from build123d import *

# Parameters (mm, degrees)
SKETCH_1_W               = 25
SKETCH_1_H               = 10
EXTRUDE_1_DEPTH          = 22.5
SKETCH_2_W               = 25
SKETCH_2_H               = 15.2
CUT_EXTRUDE_1_DEPTH      = 7.5
CUT_EXTRUDE_2_DEPTH      = 36.089172119
CUT_EXTRUDE_2_DEPTH_BACK = 36.089172119
SKETCH_4_R               = 1.03
SKETCH_5_W               = 25
SKETCH_5_H               = 4.5
EXTRUDE_2_DEPTH          = 20
SKETCH_6_W               = 11
SKETCH_6_H               = 2
CUT_EXTRUDE_3_DEPTH      = 4.5
EXTRUDE_3_DEPTH          = 3.5
SKETCH_16_R              = 9
EXTRUDE_4_DEPTH          = 6
FILLET_1_R               = 3
CUT_EXTRUDE_4_REACH      = 94.322
SKETCH_17_R              = 1.1
SKETCH_19_W              = 13
SKETCH_19_H              = 15.1
CUT_EXTRUDE_5_DEPTH      = 10
EXTRUDE_5_REACH          = 95.01
CUT_EXTRUDE_6_REACH      = 96.037
SKETCH_22_W              = 7
SKETCH_22_H              = 5
FILLET_3_R               = 2


with BuildPart() as part:
    # 草图1 → 凸台-拉伸1 (new body)
    with BuildSketch(Plane(origin=(0, 0, 0), x_dir=(1, 0, 0), z_dir=(0, 1, 0))):
        with Locations((12.5, -5)):
            Rectangle(SKETCH_1_W, SKETCH_1_H)
    extrude(amount=EXTRUDE_1_DEPTH)

    # 草图2 → 切除-拉伸1 (cut)
    with BuildSketch(Plane.XY.offset(10)):
        with Locations((12.5, 10.5)):
            Rectangle(SKETCH_2_W, SKETCH_2_H)
    extrude(amount=-CUT_EXTRUDE_1_DEPTH, mode=Mode.SUBTRACT)

    # 草图4 → 切除-拉伸2 (cut, two sides: drawn at the far end of the back side and taken through both)
    with BuildSketch(Plane(origin=(0, 22.5, 0), x_dir=(1, 0, 0), z_dir=(0, 1, 0)).offset(-CUT_EXTRUDE_2_DEPTH_BACK)):
        with Locations(Location((12.5, -5.7, 0), (0, 0, 270))):
            Circle(SKETCH_4_R)
        with Locations(Location((19.5, -5.7, 0), (0, 0, 270))):
            Circle(SKETCH_4_R)
        with Locations(Location((5.5, -5.7, 0), (0, 0, 270))):
            Circle(SKETCH_4_R)
    extrude(amount=CUT_EXTRUDE_2_DEPTH + CUT_EXTRUDE_2_DEPTH_BACK, mode=Mode.SUBTRACT)

    # 草图5 → 凸台-拉伸2 (add)
    with BuildSketch(Plane(origin=(0, 0, 0), x_dir=(-1, 0, 0), z_dir=(0, 0, -1))):
        with Locations((-12.5, 20.25)):
            Rectangle(SKETCH_5_W, SKETCH_5_H)
    extrude(amount=EXTRUDE_2_DEPTH)

    # 草图6 → 切除-拉伸3 (cut)
    with BuildSketch(Plane(origin=(0, 22.5, 0), x_dir=(1, 0, 0), z_dir=(0, 1, 0))):
        with Locations((12.5, 16)):
            Rectangle(SKETCH_6_W, SKETCH_6_H)
        with Locations((12.5, 4)):
            Rectangle(SKETCH_6_W, SKETCH_6_H)
    extrude(amount=-CUT_EXTRUDE_3_DEPTH, mode=Mode.SUBTRACT)

    # 草图15 → 凸台-拉伸3 (add)
    with BuildSketch(Plane(origin=(0, 22.5, 0), x_dir=(1, 0, 0), z_dir=(0, 1, 0))):
        Polygon((25, -2.5), (50, 11.93375673), (75, -2.5), (75, 17.5), (49.967235844, 31.914840335), (25, 17.5), align=None)
    extrude(amount=-EXTRUDE_3_DEPTH)

    # 草图16 → 凸台-拉伸4 (add)
    with BuildSketch(Plane.XZ.offset(-19)):
        with Locations(Location((75.52146997, -8.282050808, 0), (0, 0, 270))):
            Circle(SKETCH_16_R)
    extrude(amount=-EXTRUDE_4_DEPTH)

    # 圆角1
    # the kernel refuses this fillet: 3 mm, written as the material it adds along each edge
    with BuildSketch(Plane(origin=(50, 22.5, -11.93375673), x_dir=(-0.8660254037844394, 0, 0.4999999999999987), z_dir=(0, -1, 0))) as fillet_1_piece_1:
        with BuildLine():
            CenterArc((FILLET_1_R * 0.57735026919, -FILLET_1_R), FILLET_1_R, 90, 60)
            Line((-FILLET_1_R * 0.288675134595, -FILLET_1_R * 0.5), (-FILLET_1_R * 0.305995642671, -FILLET_1_R * 0.49))
            Line((-FILLET_1_R * 0.305995642671, -FILLET_1_R * 0.49), (-FILLET_1_R * 0.0115470053838, FILLET_1_R * 0.02))
            Line((-FILLET_1_R * 0.0115470053838, FILLET_1_R * 0.02), (FILLET_1_R * 0.57735026919, FILLET_1_R * 0.02))
            Line((FILLET_1_R * 0.57735026919, FILLET_1_R * 0.02), (FILLET_1_R * 0.57735026919, 0))
        make_face()
    extrude(amount=3.5)
    with BuildSketch(Plane(origin=(25, 22.5, -17.5), x_dir=(0, 0, -1), z_dir=(0, -1, 0))) as fillet_1_piece_2:
        with BuildLine():
            CenterArc((4.663812226, 2.077959733), FILLET_1_R, 150, 73.840504848)
            Line((2.065736015, 3.577959733), (2.013774491, 3.607959733))
            Line((2.013774491, 3.607959733), (-0.051961524, 0.03))
            Line((-0.051961524, 0.03), (0, -0.06))
            ThreePointArc((0, -0.06), (1.25, -0.06), (2.456723755, -0.041559195))
            Line((2.456723755, -0.041559195), (2.5, 0))
        make_face()
    extrude(amount=3.5)
    # the kernel refuses this fillet: 3 mm, written as the material it takes off along each edge
    with BuildSketch(Plane(origin=(75, 31.321038653, 2.5), x_dir=(0, 0, -1), z_dir=(0, -1, 0))) as fillet_1_2_piece_1:
        with BuildLine():
            CenterArc((4.362283942, -1.555697425), FILLET_1_R, 148.763902171, 61.236097829)
            Line((1.764207731, -3.055697425), (1.712246206, -3.085697425))
            Line((1.712246206, -3.085697425), (-0.051961524, -0.03))
            Line((-0.051961524, -0.03), (0, 0.06))
            ThreePointArc((0, 0.06), (0.898585391, 0.06), (1.745868519, 0.031113948))
            Line((1.745868519, 0.031113948), (1.797170782, 0))
        make_face()
    extrude(amount=21.142077307, mode=Mode.SUBTRACT)

    # 草图17 → 切除-拉伸4 (cut, up to next)
    with BuildSketch(Plane.XZ.offset(-19), mode=Mode.PRIVATE) as cut_extrude_4_sk1:
        with Locations(Location((75.521469969, -14.282050811, 0), (0, 0, 270))):
            Circle(SKETCH_17_R)
    cut_extrude_4_tool1 = extrude(cut_extrude_4_sk1.sketch, amount=-CUT_EXTRUDE_4_REACH, mode=Mode.PRIVATE) & part.part
    # 草图17 → 切除-拉伸4 (cut, up to next)
    with BuildSketch(Plane.XZ.offset(-19), mode=Mode.PRIVATE) as cut_extrude_4_sk2:
        with Locations(Location((75.521469969, -2.282050808, 0), (0, 0, 270))):
            Circle(SKETCH_17_R)
    cut_extrude_4_tool2 = extrude(cut_extrude_4_sk2.sketch, amount=-CUT_EXTRUDE_4_REACH, mode=Mode.PRIVATE) & part.part
    # 草图17 → 切除-拉伸4 (cut, up to next)
    with BuildSketch(Plane.XZ.offset(-19), mode=Mode.PRIVATE) as cut_extrude_4_sk3:
        with Locations(Location((69.521469967, -8.282050809, 0), (0, 0, 270))):
            Circle(SKETCH_17_R)
    cut_extrude_4_tool3 = extrude(cut_extrude_4_sk3.sketch, amount=-CUT_EXTRUDE_4_REACH, mode=Mode.PRIVATE) & part.part
    # 草图17 → 切除-拉伸4 (cut, up to next)
    with BuildSketch(Plane.XZ.offset(-19), mode=Mode.PRIVATE) as cut_extrude_4_sk4:
        with Locations(Location((81.52146997, -8.282050809, 0), (0, 0, 270))):
            Circle(SKETCH_17_R)
    cut_extrude_4_tool4 = extrude(cut_extrude_4_sk4.sketch, amount=-CUT_EXTRUDE_4_REACH, mode=Mode.PRIVATE) & part.part
    add(cut_extrude_4_tool1.solids().sort_by_distance((75.52147, 19, -14.282051))[0], mode=Mode.SUBTRACT)
    add(cut_extrude_4_tool2.solids().sort_by_distance((75.52147, 19, -2.282051))[0], mode=Mode.SUBTRACT)
    add(cut_extrude_4_tool3.solids().sort_by_distance((69.52147, 19, -8.282051))[0], mode=Mode.SUBTRACT)
    add(cut_extrude_4_tool4.solids().sort_by_distance((81.52147, 19, -8.282051))[0], mode=Mode.SUBTRACT)

    # 草图19 → 切除-拉伸5 (cut)
    with BuildSketch(Plane(origin=(0, 0, 0), x_dir=(-1, 0, 0), z_dir=(0, 0, -1))):
        with Locations((-18.5, 10.45)):
            Rectangle(SKETCH_19_W, SKETCH_19_H)
    extrude(amount=-CUT_EXTRUDE_5_DEPTH, mode=Mode.SUBTRACT)

    # 凸台-拉伸5: up to this face of the body (flat: up to its plane)
    extrude_5_end = Plane(part.part.faces().sort_by_distance((53.082748758, 19, -14.052317246))[0])
    # 草图21 → 凸台-拉伸5 (add, up to the picked face)
    with BuildSketch(Plane(origin=(0, 2.9, 0), x_dir=(1, 0, 0), z_dir=(0, 1, 0)), mode=Mode.PRIVATE) as extrude_5_sk1:
        Polygon((12, -2.5), (12, 0), (30.793852416, 6.840402867), (31.597336928, 4.632847313), align=None)
    extrude_5_tool1 = split(extrude(extrude_5_sk1.sketch, amount=EXTRUDE_5_REACH, mode=Mode.PRIVATE), bisect_by=extrude_5_end, keep=Keep.BOTH, mode=Mode.PRIVATE)
    add(extrude_5_tool1.solids().sort_by(Axis((21.599199, 2.9, -2.235102), (0, 1, 0)))[0])

    # 草图22 → 切除-拉伸6 (cut, up to next)
    with BuildSketch(Plane(origin=(2.207217853, 0, 6.064281212), x_dir=(0.9396926207859104, 0, -0.3420201433256632), z_dir=(0.3420201433256632, 0, 0.9396926207859104)), mode=Mode.PRIVATE) as cut_extrude_6_sk1:
        with Locations((27.776311449, 5.4)):
            Rectangle(SKETCH_22_W, SKETCH_22_H)
    cut_extrude_6_tool1 = extrude(cut_extrude_6_sk1.sketch, amount=-CUT_EXTRUDE_6_REACH, mode=Mode.PRIVATE) & part.part
    add(cut_extrude_6_tool1.solids().sort_by_distance((28.308413, 5.4, -3.435777))[0], mode=Mode.SUBTRACT)

    # 圆角3
    fillet_3_edges = [part.edges().sort_by_distance(p)[0] for p in [
        (31.195594672, 7.9, -5.73662509),
        (24.617746326, 2.9, -3.342484086),
        (24.617746326, 7.9, -3.342484086),
    ]]
    fillet(fillet_3_edges, radius=FILLET_3_R)


solid = part.part
Could you check a few things on this model? Use its own coordinates, in mm. A direction names the side the tool comes from. Give positions to 0.01 mm unless a question says otherwise; leave off trailing zeros. Write each loop counter-clockwise with the first axis right and the second up, starting at its lowest first coordinate (ties: lowest second). Pieces come first, ordered by that corner, then holes. Notation, with made-up numbers: (-8.75, 76.25) - (25.25, 76.25) arc R19 ccw to (25.25, 99.25) - close; hole circle Ø8 at (-11.75, 31). An arc over 180 degrees is marked (long way). Use CSV: the item, a comma, the result in double quotes. Start each with the question number.
Item 1: If I drill on line 1 along X through (y, z) = (19.2, 5.7); line 2 along Z through (x, y) = (5.5, 1.2); line 3 along Z through (x, y) = (19.5, 19.85), over which ranges is the centre line in solid material (lowest first)?
Item 2: I want a section at B-B, the plane z = 5.7. Give the number of separate pieces and of enclosed holes in the cut face, then the cut area to 3 significant figures.
Item 3: If we mould it in two halves opening along Z, with no side actions, what happens to faces 4 (the face through (73.499, 20.774, 1.137)), 5 (the face through (82.612, 21.958, -8.139)), 6 (the face through (12, 0, 4))? For each: pulls with the +Z half, pulls with the -Z half, needs draft (parallel to the pull), parting line crosses it, or undercut.
Item 4: For faces 1 (the face through (20, 18, 1)), 2 (the face through (7, 7, 0)), 3 (the face through (7, 20, -4)), which set-ups out of +Z, -Z, +X, -X, +Y, -Y let a thin tool reach every point of the face, with its end or its side?
Item 5: I want a section at A-A, the plane x = 5.5. Please give me the cut outline in (y, z).
Item 6: I want a section at C-C, the plane x = 21.5. Please give me the cut outline in (y, z).
Item 7: I want a section at D-D, the plane z = -25.5. Please give me the cut outline in (x, y).
Item 8: I'm going to push flat-ended pins straight in: pin 1 (2.5 mm diameter, centred on x = 19.5, z = 5.7, fed in from +Y); pin 2 (5.5 mm diameter, centred on x = 18.5, y = 9.5, fed in from -Z); pin 3 (1.2 mm diameter, centred on x = 5.5, z = 5.7, fed in from +Y); pin 4 (0.5 mm diameter, centred on y = 18.5, z = -15.5, fed in from +X). Where does each tip first touch, or does it pass through?
Findings:
1,line 1,"x = 0 to 4.47, 6.53 to 11.47, 13.53 to 18.47, 20.53 to 25"
1,line 2,"z = 0 to 4.67, 6.73 to 10"
1,line 3,"z = -20 to 4.67, 6.73 to 10"
2,separate pieces,"8"
2,enclosed holes,"0"
2,area,"137 mm2"
3,face 4,"pulls with the +Z half"
3,face 5,"undercut"
3,face 6,"needs draft"
4,face 1,"+Z, +X"
4,face 2,"-Z, -X, -Y"
4,face 3,"+Y, -Y"
5,outline,"(0, 0) - (18, 0) - (18, -20) - (22.5, -20) - (22.5, 4.67) - (18.1, 4.67) - (18.1, 2.5) - (2.9, 2.5) - (2.9, 4.67) - (0, 4.67) - close; (0, 6.73) - (2.9, 6.73) - (2.9, 10) - (0, 10) - close; (18.1, 6.73) - (22.5, 6.73) - (22.5, 10) - (18.1, 10) - close"
6,outline,"(0, 0) - (2.9, 0) - (2.9, 10) - (0, 10) - close; (2.9, -3.46) - (18, -3.46) - (18, -20) - (22.5, -20) - (22.5, 10) - (18.1, 10) - (18.1, 2.5) - (18, 2.5) - (18, -0.96) - (2.9, -0.96) - close"
7,outline,"(38.86, 19) - (61.11, 19) - (61.11, 22.5) - (38.86, 22.5) - close"
8,pin 1,"stops at y = 22.5"
8,pin 2,"stops at z = -3.37"
8,pin 3,"passes through"
8,pin 4,"stops at x = 25"
